The listing builds one solid part. Answer for the finished solid, in the listing's coordinates (mm). A direction names the side the tool comes from. Give positions to 0.01 mm unless a question says otherwise; leave off trailing zeros. Write each loop counter-clockwise with the first axis right and the second up, starting at its lowest first coordinate (ties: lowest second). Pieces come first, ordered by that corner, then holes. Notation, with made-up numbers: (-3, 8.5) -> (44, 8.5) arc R27 cw to (44, 42.5) -> close; hole circle Ø8 at (0.25, 39). An arc over 180 degrees is marked (long way). Put each result on its own line as item: value. Start each with the question number.
1) A cutting plane is placed at C-C (y = 97). Write down the section's boundary in (x, z), then the cut area to 3 significant figures.
2) A cutting plane is placed at B-B (x = -20). Write down the section's boundary in (y, z), then the cut area to 3 significant figures.
3) For faces 1 (the flat face through (74, 5, -5)), 2 (the flat face through (150, 74, -7)), 3 (the flat face through (1, 145, 49)), 4 (the flat face through (150, 75, 201)), 5 (the flat face through (0, 75, 201)), determine the directions among +Z, -Z, +X, -X, +Y, -Y from which every point of the face is accessible in a straight line to the end or side of a thin tool.
4) A cutting plane is placed at D-D (z = 87). Write down the section's boundary in (x, y).
5) A cutting plane is placed at A-A (z = 0). Give the number of separate pieces and of enclosed holes in the cut face, then the cut area to 3 significant figures.
6) Flat-ended cylindrical pins translate along their axes: pin 1 Ø1.5 at (y, z) = (3.5, 90) entering from -X; pin 2 Ø4 at (x, y) = (-27, 148) entering from +Z; pin 3 Ø6 at (y, z) = (105.5, -0.5) entering from +X. Find the tip coordinate at first contact, or state that the pin passes through.
7) For a pull along Y with two mould halves and no side action, classify faces 6 (the flat face through (74, 76, -15)), 7 (the flat face through (149, 5, 49)), 8 (the flat face through (77, 76, -20)), 9 (the flat face through (76, 0, 1)) as released by +Y, released by -Y, zero draft, split by the parting line, or undercut.
8) Find the intervals of material crossed by line 1 along X through (y, z) = (148, 0); line 2 along Y through (x, z) = (149, 57); line 3 along Z through (x, y) = (40.5, 114), in increasing order. Write a range as from..to.
from build123d import *

# Parameters (mm, degrees)
SKETCH_1_W                  = 150
SKETCH_1_H                  = 150
SKETCH_1_W_2                = 140
SKETCH_1_H_2                = 140
EXTRUDE_2_DEPTH             = 5
SKETCH_1_4_W                = 40
SKETCH_1_4_H                = 5
EXTRUDE_3_DEPTH             = 20
SKETCH_2_R                  = 12.5
CUT_EXTRUDE_1_DEPTH         = 243.89915603
PATTERN_LINEAR_1_COUNT      = 2
PATTERN_LINEAR_1_PITCH      = 190
SKETCH_4_W                  = 5
SKETCH_4_H                  = 5
EXTRUDE_5_DEPTH             = 200
PATTERN_LINEAR_2_COUNT      = 2
PATTERN_LINEAR_2_PITCH      = 145
PATTERN_LINEAR_2_COUNT_DIR2 = 2
PATTERN_LINEAR_2_PITCH_DIR2 = 145
PATTERN_LINEAR_3_COUNT      = 2
PATTERN_LINEAR_3_PITCH      = 200
SKETCH_5_W                  = 150
SKETCH_5_H                  = 150
EXTRUDE_6_DEPTH             = 20
SKETCH_7_W                  = 140
SKETCH_7_H                  = 140
CUT_EXTRUDE_3_DEPTH         = 15


with BuildPart() as part:
    # Sketch 1 → Extrude 2 (new body)
    with BuildSketch(Plane.XY):
        with Locations((75, 75)):
            Rectangle(SKETCH_1_W, SKETCH_1_H)
        with Locations((75, 75)):
            Rectangle(SKETCH_1_W_2, SKETCH_1_H_2, mode=Mode.SUBTRACT)
    extrude_2 = extrude(amount=EXTRUDE_2_DEPTH)

    # Sketch 1_4 → Extrude 3 (add, symmetric)
    with BuildSketch(Plane.XY):
        with Locations((170, 147.5)):
            Rectangle(SKETCH_1_4_W, SKETCH_1_4_H)
        with Locations((-20, 147.5)):
            Rectangle(SKETCH_1_4_W, SKETCH_1_4_H)
        with Locations((170, 2.5)):
            Rectangle(SKETCH_1_4_W, SKETCH_1_4_H)
        with Locations((-20, 2.5)):
            Rectangle(SKETCH_1_4_W, SKETCH_1_4_H)
    extrude(amount=EXTRUDE_3_DEPTH, both=True)

    # Sketch 2 → Cut-Extrude 1 (cut, through all)
    with BuildSketch(Plane.XZ):
        with Locations(Location((-20, 0, 0), (0, 0, 270))):
            Circle(SKETCH_2_R)
    cut_extrude_1 = extrude(amount=-CUT_EXTRUDE_1_DEPTH, mode=Mode.SUBTRACT)

    # Pattern Linear 1: Cut-Extrude 1 ×2
    with Locations(*[(i * PATTERN_LINEAR_1_PITCH, 0, 0) for i in range(1, PATTERN_LINEAR_1_COUNT)]):
        add(cut_extrude_1, mode=Mode.SUBTRACT)

    # Sketch 4 → Extrude 5 (add)
    with BuildSketch(Plane.XY.offset(5)):
        with Locations((147.5, 2.5)):
            Rectangle(SKETCH_4_W, SKETCH_4_H)
    extrude_5 = extrude(amount=EXTRUDE_5_DEPTH)

    # Pattern Linear 2: Extrude 5 2 × 2
    with Locations(*[(-j * PATTERN_LINEAR_2_PITCH_DIR2, i * PATTERN_LINEAR_2_PITCH, 0) for i in range(PATTERN_LINEAR_2_COUNT) for j in range(PATTERN_LINEAR_2_COUNT_DIR2) if (i, j) != (0, 0)]):
        add(extrude_5)

    # Pattern Linear 3: Extrude 2 ×2
    with Locations(*[(0, 0, i * PATTERN_LINEAR_3_PITCH) for i in range(1, PATTERN_LINEAR_3_COUNT)]):
        add(extrude_2)

    # Sketch 5 → Extrude 6 (add)
    with BuildSketch(Plane(origin=(0, 0, 0), x_dir=(-1, 0, 0), z_dir=(0, 0, -1))):
        with Locations((-75, 75)):
            Rectangle(SKETCH_5_W, SKETCH_5_H)
    extrude(amount=EXTRUDE_6_DEPTH)

    # Sketch 7 → Cut-Extrude 3 (cut)
    with BuildSketch(Plane.XY):
        with Locations((75, 75)):
            Rectangle(SKETCH_7_W, SKETCH_7_H)
    extrude(amount=-CUT_EXTRUDE_3_DEPTH, mode=Mode.SUBTRACT)


solid = part.part
Reply:
1. outline: (0, -20) -> (150, -20) -> (150, 5) -> (145, 5) -> (145, -15) -> (5, -15) -> (5, 5) -> (0, 5) -> close; (0, 200) -> (5, 200) -> (5, 205) -> (0, 205) -> close; (145, 200) -> (150, 200) -> (150, 205) -> (145, 205) -> close
1. area: 1,000 mm2
2. outline: (0, -20) -> (5, -20) -> (5, -12.5) -> (0, -12.5) -> close; (0, 12.5) -> (5, 12.5) -> (5, 20) -> (0, 20) -> close; (145, -20) -> (150, -20) -> (150, -12.5) -> (145, -12.5) -> close; (145, 12.5) -> (150, 12.5) -> (150, 20) -> (145, 20) -> close
2. area: 150 mm2
3. face 1: +Z
3. face 2: +Z, -Z, +X
3. face 3: -X
3. face 4: +Z, +X, +Y, -Y
3. face 5: +Z, -X, +Y, -Y
4. outline: (0, 0) -> (5, 0) -> (5, 5) -> (0, 5) -> close; (0, 145) -> (5, 145) -> (5, 150) -> (0, 150) -> close; (145, 0) -> (150, 0) -> (150, 5) -> (145, 5) -> close; (145, 145) -> (150, 145) -> (150, 150) -> (145, 150) -> close
5. separate pieces: 5
5. enclosed holes: 1
5. area: 3,200 mm2
6. pin 1: stops at x = 0
6. pin 2: stops at z = 20
6. pin 3: stops at x = 150
7. face 6: undercut
7. face 7: undercut
7. face 8: zero draft
7. face 9: released by -Y
8. line 1: x = -40..-32.5, -7.5..157.5, 182.5..190
8. line 2: y = 0..5, 145..150
8. line 3: z = -20..-15
